```python
from build123d import *

# Parameters (mm, degrees)
F1_DEPTH = 8


with BuildPart() as f1:
    # F0 (on Front) → F1 (new body)
    with BuildSketch(Plane.XZ):
        Polygon((-47.1591800451, -3.9871255867), (-47.1591800451, -46.8671731651), (-3.0660768971, -46.8671731651), (-3.0660768971, -42.9581068456), (-43.1017912924, -42.9581068456), (-43.1017912924, -3.9871255867), align=None)
        Polygon((-54.3611483469, -3.9871255867), (-47.1591800451, -3.9871255867), (-43.1017912924, -3.9871255867), (-43.1017912924, -2.1041460184), (-54.3611483469, -1.8037535483), align=None)
        with BuildLine():
            Line((-43.1017912924, -42.9581068456), (-3.0660768971, -42.9581068456))
            Line((-3.0660768971, -42.9581068456), (-3.0660768971, -36.9308893154))
            ThreePointArc((-3.0660768971, -36.9308893154), (-25.8747586881, -26.5290081986), (-36.8428316328, -3.9871255867))
            Line((-36.8428316328, -3.9871255867), (-43.1017912924, -3.9871255867))
            Line((-43.1017912924, -3.9871255867), (-43.1017912924, -42.9581068456))
        make_face()
        with BuildLine():
            Line((-43.1017912924, -2.1041460184), (-43.1017912924, -3.9871255867))
            Line((-43.1017912924, -3.9871255867), (-36.8428316328, -3.9871255867))
            ThreePointArc((-36.8428316328, -3.9871255867), (-36.9256932446, -3.12803318), (-36.9885254852, -2.2672440539))
            Line((-36.9885254852, -2.2672440539), (-43.1017912924, -2.1041460184))
        make_face()
        with BuildLine():
            ThreePointArc((-36.8428316328, -3.9871255867), (-25.8747586881, -26.5290081986), (-3.0660768971, -36.9308893154))
            Line((-3.0660768971, -36.9308893154), (-3.0660768971, -34.3354971844))
            ThreePointArc((-3.0660768971, -34.3354971844), (-24.0459151958, -24.7006306971), (-34.2407655288, -3.9871255867))
            Line((-34.2407655288, -3.9871255867), (-36.8428316328, -3.9871255867))
        make_face()
        with BuildLine():
            Line((-3.0660768971, -34.3354971844), (-3.0660768971, -36.9308893154))
            ThreePointArc((-3.0660768971, -36.9308893154), (-2.0633689571, -37.0004583987), (-1.0591430979, -37.0428080613))
            Line((-1.0591430979, -37.0428080613), (-1.1211578882, -34.4538851137))
            ThreePointArc((-1.1211578882, -34.4538851137), (-2.0944540368, -34.4084358367), (-3.0660768971, -34.3354971844))
        make_face()
        with BuildLine():
            Line((-43.1017912924, 0.534063729), (-43.1017912924, -2.1041460184))
            Line((-43.1017912924, -2.1041460184), (-36.9885254852, -2.2672440539))
            ThreePointArc((-36.9885254852, -2.2672440539), (-37.0477983113, -0.867210155), (-37.0540981418, 0.534063729))
            Line((-37.0540981418, 0.534063729), (-43.1017912924, 0.534063729))
        make_face()
        with BuildLine():
            Line((-1.1211578882, -34.4538851137), (-1.0591430979, -37.0428080613))
            ThreePointArc((-1.0591430979, -37.0428080613), (0.3177187709, -37.0565846774), (1.6941420035, -37.0192017207))
            Line((1.6941420035, -37.0192017207), (1.6941420035, -34.4304672828))
            ThreePointArc((1.6941420035, -34.4304672828), (0.2867312292, -34.4709294862), (-1.1211578882, -34.4538851137))
        make_face()
        with BuildLine():
            Line((-43.1017912924, 1.8888709601), (-43.1017912924, 0.534063729))
            Line((-43.1017912924, 0.534063729), (-37.0540981418, 0.534063729))
            ThreePointArc((-37.0540981418, 0.534063729), (-37.0381326331, 1.2116700136), (-37.0097768119, 1.8888709601))
            Line((-37.0097768119, 1.8888709601), (-43.1017912924, 1.8888709601))
        make_face()
        with BuildLine():
            ThreePointArc((3.3580851741, -36.9054830226), (2.5267534207, -36.9717044551), (1.6941420035, -37.0192017207))
            Line((1.6941420035, -37.0192017207), (1.6941420035, -55.0743453205))
            Line((1.6941420035, -55.0743453205), (3.3580851741, -55.0743453205))
            Line((3.3580851741, -55.0743453205), (3.3580851741, -46.8671731651))
            Line((3.3580851741, -46.8671731651), (3.3580851741, -42.7945544943))
            Line((3.3580851741, -42.7945544943), (3.3580851741, -36.9054830226))
        make_face()
        with BuildLine():
            Line((1.6941420035, -34.4304672828), (1.6941420035, -37.0192017207))
            ThreePointArc((1.6941420035, -37.0192017207), (2.5267534207, -36.9717044551), (3.3580851741, -36.9054830226))
            Line((3.3580851741, -36.9054830226), (3.3580851741, -34.3081689748))
            ThreePointArc((3.3580851741, -34.3081689748), (2.5268535934, -34.3793863435), (1.6941420035, -34.4304672828))
        make_face()
        Polygon((-47.1591800451, 1.8888709601), (-43.1017912924, 1.8888709601), (-43.1017912924, 41.1945804954), (-43.1017912924, 41.6629081592), (-3.0660768971, 41.6629081592), (-3.0660768971, 45.4071350396), (-47.1591800451, 45.4071350396), align=None)
        with BuildLine():
            Line((-43.1017912924, 41.1945804954), (-43.1017912924, 1.8888709601))
            Line((-43.1017912924, 1.8888709601), (-37.0097768119, 1.8888709601))
            ThreePointArc((-37.0097768119, 1.8888709601), (-26.6177436164, 25.7834663678), (-3.0660768971, 36.9308893154))
            Line((-3.0660768971, 36.9308893154), (-3.0660768971, 41.6629081592))
            Line((-3.0660768971, 41.6629081592), (-43.1017912924, 41.6629081592))
            Line((-43.1017912924, 41.6629081592), (-43.1017912924, 41.1945804954))
        make_face()
        with BuildLine():
            ThreePointArc((36.8810945474, -3.6161136812), (26.1121317389, -26.295398632), (3.3580851741, -36.9054830226))
            Line((3.3580851741, -36.9054830226), (3.3580851741, -42.7945544943))
            Line((3.3580851741, -42.7945544943), (41.5107160807, -42.9581068456))
            Line((41.5107160807, -42.9581068456), (41.5107160807, -3.876257455))
            Line((41.5107160807, -3.876257455), (36.8810945474, -3.6161136813))
        make_face()
        with BuildLine():
            Line((3.3580851741, -34.3081689748), (3.3580851741, -36.9054830226))
            ThreePointArc((3.3580851741, -36.9054830226), (26.1121317389, -26.295398632), (36.8810945474, -3.6161136812))
            Line((36.8810945474, -3.6161136813), (34.2969386269, -3.4709069795))
            ThreePointArc((34.2969386269, -3.4709069795), (24.3353526008, -24.4155239189), (3.3580851741, -34.3081689748))
        make_face()
        with BuildLine():
            Line((34.2969386269, -3.4709069795), (36.8810945474, -3.6161136813))
            ThreePointArc((36.8810945474, -3.6161136812), (36.9391000222, -2.9655189628), (36.9856296892, -2.3140029516))
            Line((36.9856296892, -2.3140029516), (34.3943685039, -2.3140029516))
            ThreePointArc((34.3943685039, -2.3140029516), (34.3505243856, -2.8928651668), (34.2969386269, -3.4709069795))
        make_face()
        with BuildLine():
            ThreePointArc((-1.0392403929, 37.0433717765), (-2.0534289831, 37.0010113724), (-3.0660768971, 36.9308893154))
            Line((-3.0660768971, 36.9308893154), (-3.0660768971, 34.3354971844))
            ThreePointArc((-3.0660768971, 34.3354971844), (-2.0535493927, 34.4109013153), (-1.0392403929, 34.4564532976))
            Line((-1.0392403929, 34.4564532976), (-1.0392403929, 37.0433717765))
        make_face()
        with BuildLine():
            Line((-3.0660768971, 41.6629081592), (-3.0660768971, 36.9308893154))
            ThreePointArc((-3.0660768971, 36.9308893154), (-2.0534289831, 37.0010113724), (-1.0392403929, 37.0433717765))
            Line((-1.0392403929, 37.0433717765), (-1.0392403929, 41.6629081592))
            Line((-1.0392403929, 41.6629081592), (-3.0660768971, 41.6629081592))
        make_face()
        with BuildLine():
            Line((34.3943685039, -2.3140029516), (36.9856296892, -2.3140029516))
            ThreePointArc((36.9856296892, -2.3140029516), (37.0398630305, -1.157566349), (37.0579466939, 0))
            ThreePointArc((37.0579466939, 0), (37.0571653007, 0.2406512887), (37.0548211541, 0.4812924287))
            Line((37.0548211541, 0.4812924287), (34.4676887508, 0.5528350755))
            ThreePointArc((34.4676887508, 0.5528350755), (34.4710136618, 0.2764264252), (34.4721219892, 0))
            ThreePointArc((34.4721219892, 0), (34.4526781343, -1.1576544459), (34.3943685039, -2.3140029516))
        make_face()
        with BuildLine():
            ThreePointArc((37.0579466939, 0), (37.0398630305, -1.157566349), (36.9856296892, -2.3140029516))
            Line((36.9856296892, -2.3140029516), (54.4263494667, -2.3140029516))
            Line((54.4263494667, -2.3140029516), (54.4593664818, 0))
            Line((54.4593664818, 0), (45.8812378347, 0.2372132275))
            Line((45.8812378347, 0.2372132275), (37.0548211541, 0.4812924287))
            ThreePointArc((37.0548211541, 0.4812924287), (37.0571653007, 0.2406512887), (37.0579466939, 0))
        make_face()
        with BuildLine():
            ThreePointArc((2.8755131643, 36.9462154653), (0.919420611, 37.0465393648), (-1.0392403929, 37.0433717765))
            Line((-1.0392403929, 37.0433717765), (-1.0392403929, 34.4564532976))
            ThreePointArc((-1.0392403929, 34.4564532976), (0.9196211301, 34.4598533284), (2.8755131643, 34.351981289))
            Line((2.8755131643, 34.351981289), (2.8755131643, 36.9462154653))
        make_face()
        Polygon((54.4593664818, 0), (54.4263494667, -2.3140029516), (54.3960799696, -4.4354456477), (54.4593664818, -4.4354456477), align=None)
        with BuildLine():
            ThreePointArc((4.2341067456, 36.8152652202), (3.5554128885, 36.886995708), (2.8755131643, 36.9462154653))
            Line((2.8755131643, 36.9462154653), (2.8755131643, 34.351981289))
            ThreePointArc((2.8755131643, 34.351981289), (3.555507773, 34.2882714484), (4.2341067456, 34.2111025035))
            Line((4.2341067456, 34.2111025035), (4.2341067456, 36.8152652202))
        make_face()
        with BuildLine():
            ThreePointArc((37.0162491765, 1.7574726371), (37.0410316266, 1.119548661), (37.0548211541, 0.4812924287))
            Line((37.0548211541, 0.4812924287), (45.8812378347, 0.2372132275))
            Line((45.8812378347, 0.2372132275), (45.8812378347, 1.7574726371))
            Line((45.8812378347, 1.7574726371), (41.5107160807, 1.7574726371))
            Line((41.5107160807, 1.7574726371), (37.0162491765, 1.7574726371))
        make_face()
        Polygon((45.8812378347, 0.2372132275), (54.4593664818, 0), (54.4593664818, 1.7574726371), (45.8812378347, 1.7574726371), align=None)
        with BuildLine():
            ThreePointArc((37.0162491765, 1.7574726371), (27.0676960808, 25.3106942229), (4.2341067456, 36.8152652202))
            Line((4.2341067456, 36.8152652202), (4.2341067456, 34.2111025035))
            ThreePointArc((4.2341067456, 34.2111025035), (25.2385711785, 23.4806669264), (34.427292725, 1.7574726371))
            Line((34.427292725, 1.7574726371), (37.0162491765, 1.7574726371))
        make_face()
        with BuildLine():
            Line((4.2341067456, 41.2198267877), (4.2341067456, 36.8152652202))
            ThreePointArc((4.2341067456, 36.8152652202), (27.0676960808, 25.3106942229), (37.0162491765, 1.7574726371))
            Line((37.0162491765, 1.7574726371), (41.5107160807, 1.7574726371))
            Line((41.5107160807, 1.7574726371), (41.5107160807, 41.2198267877))
            Line((41.5107160807, 41.2198267877), (4.2341067456, 41.2198267877))
        make_face()
        Polygon((4.2341067456, 45.9911525249), (4.2341067456, 41.2198267877), (41.5107160807, 41.2198267877), (41.5107160807, 1.7574726371), (45.8812378347, 1.7574726371), (45.8812378347, 45.9911525249), align=None)
    extrude(amount=F1_DEPTH)


solid = f1.part
```
Work out the finished part from the listing and answer in its coordinate system (mm). A direction names the side the tool comes from. Give positions to 0.01 mm unless a question says otherwise; leave off trailing zeros. Write each loop counter-clockwise with the first axis right and the second up, starting at its lowest first coordinate (ties: lowest second). Pieces come first, ordered by that corner, then holes.
(1) The part is cut by section A-A on z = -41. Write down the section's boundary in (x, y), plus the area to 3 significant figures.
Final values:
outline: (-47.16, -8) - (-3.07, -8) - (-3.07, 0) - (-47.16, 0) - close; (1.69, -8) - (41.51, -8) - (41.51, 0) - (1.69, 0) - close
area: 671 mm2
(2) The part is cut by section C-C on x = 44.5. Write down the section's boundary in (y, z), plus the area to 3 significant figures.
Final values:
outline: (-8, -2.31) - (0, -2.31) - (0, 45.99) - (-8, 45.99) - close
area: 386 mm2
(3) The part is cut by section B-B on x = 19.5. Write down the section's boundary in (y, z), plus the area to 3 significant figures.
Final values:
outline: (-8, -42.86) - (0, -42.86) - (0, -28.43) - (-8, -28.43) - close; (-8, 28.43) - (0, 28.43) - (0, 45.99) - (-8, 45.99) - close
area: 256 mm2
(4) The mould has two halves that part along Z. Classify faces 1 (the flat face through (3.358, -4, -49)), 2 (the flat face through (-45, -4, 1.889)), 3 (the flat face through (-25, -4, -46.867)): pulls with the +Z half, pulls with the -Z half, needs draft (parallel to the pull), parting line crosses it, or undercut.
Final values:
face 1: needs draft
face 2: undercut
face 3: pulls with the -Z half
(5) Flat-ended cylindrical pins translate along their axes: pin 1 Ø2 at (x, y) = (-18.5, -6.5) entering from +Z; pin 2 Ø2.5 at (y, z) = (-6, -43.5) entering from -X; pin 3 Ø2.5 at (y, z) = (-3, 38.5) entering from +X. Find the tip coordinate at first contact, or state that the pin passes through.
Final values:
pin 1: stops at z = 45.41
pin 2: stops at x = -47.16
pin 3: stops at x = 45.88
(6) Straight lines are drawn through the part: line 1 (X direction, y = -4.5, z = 39); line 2 (X direction, y = -5.25, z = -50); line 3 (X direction, y = -7, z = -4.5). For each, find the intervals that lie inside material, in ascending order.
Final values:
line 1: x = -47.16 to -1.04, 4.23 to 45.88
line 2: x = 1.69 to 3.36
line 3: x = -47.16 to -34.18, 34.18 to 41.51
(7) Which of the six approach directions +Z, -Z, +X, -X, +Y, -Y give full straight-line access (tool end or side, diameter ignored) to faces 4 (the flat face through (36, -4, 1.757)), 5 (the flat face through (-3.066, -4, -42)), 6 (the flat face through (-1.039, -4, 39)), 7 (the flat face through (-47.159, -4, 24))?
Final values:
face 4: +Y, -Y
face 5: -Z, +Y, -Y
face 6: +Z, +Y, -Y
face 7: +Z, -X, +Y, -Y
